Autodesk Inventor part; units mm, degrees
ref_plane "YZ Plane" through (0, 0, 0) normal (1, 0, 0) x (0, 1, 0)
ref_plane "XZ Plane" through (0, 0, 0) normal (0, 1, 0) x (-1, 0, 0)
ref_plane "XY Plane" through (0, 0, 0) normal (0, 0, 1) x (1, 0, 0)
sketch "Sketch1" plane through (0, 0, 0) normal (0, 0, 1) x (1, 0, 0)
  line L0 (0, 0) -> (200, 0)
  line L1 (200, 0) -> (200, 80)
  line L2 (200, 80) -> (0, 80)
  line L3 (0, 80) -> (0, 0)
  dimension "d0" = 200
  dimension "d1" = 80
extrude "Extrusion1" add sketch "Sketch1" along normal blind 3
sketch "Sketch2" plane through (0, 0, 3) normal (0, 0, 1) x (1, 0, 0)
  line L0 (0, 0) -> (0, 3)
  line L1 (0, 3) -> (40, 3)
  line L2 (40, 3) -> (40, 0)
  line L3 (0, 0) -> (200, 0)
  line L4 (40, 0) -> (80, 0)
  line L5 (80, 0) -> (80, 3)
  line L6 (80, 3) -> (120, 3)
  line L7 (120, 3) -> (120, 0)
  line L8 (120, 0) -> (160, 0)
  line L9 (160, 0) -> (160, 3)
  line L10 (160, 3) -> (200, 3)
  line L11 (0, 80) -> (0, 0)
  line L12 (0, 80) -> (0, 77)
  line L13 (0, 77) -> (40, 77)
  line L14 (40, 77) -> (40, 80)
  line L15 (0, 80) -> (200, 80)
  line L16 (40, 80) -> (80, 80)
  line L17 (80, 80) -> (80, 77)
  line L18 (80, 77) -> (120, 77)
  line L19 (120, 77) -> (120, 80)
  line L20 (120, 80) -> (160, 80)
  line L21 (160, 80) -> (160, 77)
  line L22 (160, 77) -> (200, 77)
  line L23 (200, 80) -> (0, 80)
  line L24 (0, 80) -> (0, 53.3333)
  line L25 (0, 53.3333) -> (3, 53.3333)
  line L26 (3, 53.3333) -> (3, 26.6667)
  line L27 (3, 26.6667) -> (0, 26.6667)
  line L28 (200, 53.3333) -> (197, 53.3333)
  line L29 (197, 53.3333) -> (197, 26.6667)
  line L30 (197, 26.6667) -> (200, 26.6667)
  line L31 (160, 77) -> (160, 80)
  line L32 (200, 77) -> (200, 80)
  line L33 (200, 3) -> (200, 0)
  line L34 (200, 26.6667) -> (200, 53.3333)
  dimension "d4" = 3
  dimension "d5" = 40
  dimension "d6" = 40
  dimension "d7" = 40
  dimension "d8" = 40
  dimension "d9" = 26.6667
  dimension "d10" = 3
  dimension "d11" = 26.6667
extrude "Extrusion2" cut sketch "Sketch2" against normal blind 3
properties part number "TAPA 2"
For this review, take the finished solid that the model builds, in its own axes (mm). Coordinates: 2 decimals unless noted, no trailing zeros. Loops run counter-clockwise (first coordinate to the right, second up) from the corner with the lowest first, then second, coordinate; pieces in that order, holes last. Notation, with made-up numbers: (-29, -33.75) -> (-24, -33.75) arc R23 ccw to (-24, -7.75) -> close; hole circle Ø10 at (9, -26). An arc over 180 degrees is marked (long way). Write each question's results on one line, items separated by ' | '.
Q1. Add section C-C, the plane x = 175.5. State the section outline as (y, z) points.
Taken from the geometry:
outline: (3, 0) -> (77, 0) -> (77, 3) -> (3, 3) -> close
Q2. Add section B-B, the plane y = 44. State the section outline as (x, z) points.
Taken from the geometry:
outline: (3, 0) -> (197, 0) -> (197, 3) -> (3, 3) -> close
Q3. For pin 1 Ø0.9 at (y, z) = (1, 2) entering from +X; pin 2 Ø0.9 at (x, z) = (95, 1.5) entering from -Y; pin 3 Ø0.9 at (x, z) = (29, 2) entering from +Y, all flat-tipped, find the tip position at first contact; note any pin that passes through.
Taken from the geometry:
pin 1: x = 160 | pin 2: y = 3 | pin 3: y = 77
Q4. To check wall thickness, follow line 1 along Y through (x, z) = (100, 1.75); line 2 along X through (y, z) = (47, 2.5). State the ranges of each line that lie inside material, in increasing order. Write a range as [from, to].
Taken from the geometry:
line 1: [3, 77] | line 2: [3, 197]
Q5. Add section A-A, the plane z = 2.4. State the section outline as (x, y) points.
Taken from the geometry:
outline: (0, 3) -> (40, 3) -> (40, 0) -> (80, 0) -> (80, 3) -> (120, 3) -> (120, 0) -> (160, 0) -> (160, 3) -> (200, 3) -> (200, 26.67) -> (197, 26.67) -> (197, 53.33) -> (200, 53.33) -> (200, 77) -> (160, 77) -> (160, 80) -> (120, 80) -> (120, 77) -> (80, 77) -> (80, 80) -> (40, 80) -> (40, 77) -> (0, 77) -> (0, 53.33) -> (3, 53.33) -> (3, 26.67) -> (0, 26.67) -> close
